For this review, take the finished solid that the model builds, in its own axes (mm). A direction names the side the tool comes from. Coordinates: 2 decimals unless noted, no trailing zeros. Loops run counter-clockwise (first coordinate to the right, second up) from the corner with the lowest first, then second, coordinate; pieces in that order, holes last. Notation, with made-up numbers: M 22,84 L 34,84 A12 ccw 34,104 Z; hole C 53.5,5.25 d8. An arc over 180 degrees is marked long. Put each result on its own line as item: value.
```python
from build123d import *

# Parameters (mm, degrees)
LINEAR_AUSTRAGEN_D_NN1_DEPTH = 95
VERRUNDUNG1_R                = 2
VERRUNDUNG2_R                = 1


with BuildPart() as part:
    # Skizze1 → Linear-Austragen-Dünn1 (new body)
    with BuildSketch(Plane(origin=(0, 0, 0), x_dir=(0, 0, -1), z_dir=(1, 0, 0))):
        with BuildLine():
            Line((-13.106432709, 9.177222982), (-6.228450194, 19))
            Line((-6.228450194, 19), (6.228450194, 19))
            Line((6.228450194, 19), (13.106432709, 9.177222982))
            ThreePointArc((13.106432709, 9.177222982), (0, -16), (-13.106432709, 9.177222982))
        make_face()
        with BuildLine():
            Line((-12.287280664, 8.603646545), (-5.707883144, 18))
            Line((-5.707883144, 18), (5.707883144, 18))
            Line((5.707883144, 18), (12.287280664, 8.603646545))
            ThreePointArc((12.287280664, 8.603646545), (0, -15), (-12.287280664, 8.603646545))
        make_face(mode=Mode.SUBTRACT)
    extrude(amount=LINEAR_AUSTRAGEN_D_NN1_DEPTH)

    # Verrundung1
    verrundung1_edges = [part.edges().sort_by_distance(p)[0] for p in [
        (47.5, 19, 6.228450194),
        (47.5, 19, -6.228450194),
    ]]
    fillet(verrundung1_edges, radius=VERRUNDUNG1_R)

    # Verrundung2
    verrundung2_edges = [part.edges().sort_by_distance(p)[0] for p in [
        (47.5, 18, -5.707883144),
        (47.5, 18, 5.707883144),
    ]]
    fillet(verrundung2_edges, radius=VERRUNDUNG2_R)


solid = part.part
```
(1) Tool access review of faces 1 (the cylindrical face through (48.16, 18.77, 6.12)), 2 (the flat face through (46.835, 13.151, -9.103)): name each direction out of +Z, -Z, +X, -X, +Y, -Y from which nothing blocks a thin tool from reaching the whole face with its end or side.
Determined:
face 1: +Z, +X, -X, +Y
face 2: +X, -X
(2) Wall thickness on line 1 along Z through (x, y) = (53, 0); line 2 along Y through (x, z) = (16, 13.5); line 3 along Z through (x, y) = (50, -11): over which ranges is each line inside the solid? List them lowest first. Write a range as [from, to].
Determined:
line 1: z = [-16, -15], [15, 16]
line 2: y = [-8.59, -6.54], [6.54, 8.59]
line 3: z = [-11.62, -10.2], [10.2, 11.62]
(3) Add section C-C (x = 19.5). Write out the cut boundary in (y, z).
Determined:
outline: M 9.18,-13.11 L 18.15,-6.83 A2 ccw 19,-5.19 L 19,5.19 A2 ccw 18.15,6.83 L 9.18,13.11 A16 ccw long Z; hole M 8.6,-12.29 L 17.57,-6.01 A1 ccw 18,-5.19 L 18,5.19 A1 ccw 17.57,6.01 L 8.6,12.29 A15 ccw long Z
(4) Add section B-B (z = 0). Write out the cut boundary in (x, y).
Determined:
outline: M 0,-16 L 95,-16 L 95,-15 L 0,-15 Z; M 0,18 L 95,18 L 95,19 L 0,19 Z
(5) Add section A-A (y = 0). Write out the cut boundary in (x, z).
Determined:
outline: M 0,-16 L 95,-16 L 95,-15 L 0,-15 Z; M 0,15 L 95,15 L 95,16 L 0,16 Z
(6) Draft analysis for pull direction Y (two halves, no side actions). For faces 3 (the flat face through (0, 8, 13)), 4 (the flat face through (47, 18, 0)), 5 (the flat face through (47, 19, 0)), state which applies: +Y half, -Y half, draft (parallel to the pull), parting line (faces both ways), or undercut.
Determined:
face 3: draft
face 4: undercut
face 5: +Y half
(7) For pin 1 (4 mm diameter, centred on x = 63, y = -3.5, fed in from -Z); pin 2 (1.5 mm diameter, centred on x = 68.5, z = 10.5, fed in from -Y); pin 3 (2 mm diameter, centred on x = 41, z = -5, fed in from -Y); pin 4 (4 mm diameter, centred on y = 2.5, z = 12.5, fed in from -X), all flat-tipped, find the tip position at first contact; note any pin that passes through.
Determined:
pin 1: stops at z = -15.93
pin 2: stops at y = -12.69
pin 3: stops at y = -15.49
pin 4: passes through
